Here's how the part is built. I have some questions about the finished solid (model axes, mm). Face numbers are marked on the shaded views. A direction names the side the tool comes from. Give positions to 0.01 mm unless a question says otherwise; leave off trailing zeros. Loops run counter-clockwise (first coordinate to the right, second up) from the corner with the lowest first, then second, coordinate; pieces in that order, holes last.
Q1. If we section it at D-D (z = 0): Give the number of separate pieces and of enclosed holes in the cut face, plus the area to 3 significant figures.
Q2. Will these pins go through, and if not, where does the flat tip stop? P1, Ø1.3, axis at x = 33, z = -56.5, coming from the +Y side; P2, Ø4, axis at x = -28, z = 35.5, coming from the +Y side; P3, Ø16.5, axis at x = 56.5, y = 13.5, coming from the -Z side.
Q3. If we section it at A-A (z = -35.5): Please give me the cut outline in (x, y).
Q4. We'd pull the mould along Y, two halves only. Please class the marked faces 1, 2 and 3: +Y half, -Y half, draft (parallel to the pull), parting line (faces both ways), or undercut.
Q5. For the marked faces 4, 5 and 6, which set-ups out of +Z, -Z, +X, -X, +Y, -Y let a thin tool reach every point of the face, with its end or its side?
Q6. I need wall thicknesses on line 1 (Z direction, x = 68, y = 27); line 2 (Z direction, x = -14, y = 16); line 3 (Y direction, x = 53, z = -8). Which ranges of each line are inside material? Lowest first, please.
Q7. If we section it at C-C (y = 11.5): Please give me the cut outline in (x, z), plus the area to 3 significant figures.
Q8. If we section it at B-B (x = 13): Please give me the cut outline in (y, z).
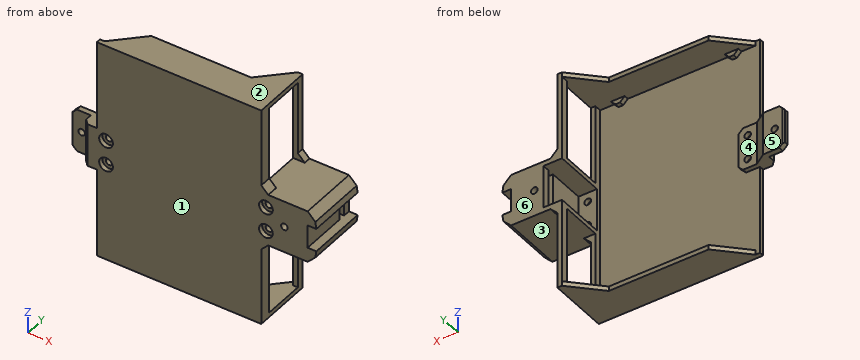
from build123d import *

# Parameters (mm, degrees)
SKETCH3_W                                       = 90.422573022
SKETCH3_H                                       = 121.412
BOSS_EXTRUDE4_DEPTH                             = 2.54
BOSS_EXTRUDE5_DEPTH                             = 30.48
CUT_EXTRUDE2_DEPTH                              = 122.412
BOSS_EXTRUDE6_DEPTH                             = 33.02
SKETCH9_W                                       = 10.16
SKETCH9_H                                       = 23.622
CUT_EXTRUDE3_DEPTH                              = 27.94
BOSS_EXTRUDE7_DEPTH                             = 2.54
SKETCH12_W                                      = 23.622
SKETCH12_H                                      = 3.81
CUT_EXTRUDE4_DEPTH                              = 10.16
SKETCH13_W                                      = 12.7
SKETCH13_H                                      = 3.81
CUT_EXTRUDE5_DEPTH                              = 13.461069207
BOSS_EXTRUDE9_REACH                             = 62.706
BOSS_EXTRUDE9_DIRECTION_2_REACH                 = 62.706
CBORE_FOR_6_PAN_HEAD_MACHINE_SCREW1_D           = 3.6576
CBORE_FOR_6_PAN_HEAD_MACHINE_SCREW1_CBORE_D     = 7.54126
CBORE_FOR_6_PAN_HEAD_MACHINE_SCREW1_CBORE_DEPTH = 2.4638
F_6_CLEARANCE_HOLE1_D                           = 3.6576
SKETCH21_W                                      = 43.815
SKETCH21_H                                      = 22.86
CUT_EXTRUDE6_DEPTH                              = 33.781069207
CHAMFER1_SIZE                                   = 2.54
CHAMFER2_SIZE                                   = 3.81
SKETCH22_W                                      = 17.78
SKETCH22_H                                      = 23.622
CUT_EXTRUDE7_DEPTH                              = 0.8
CHAMFER3_SIZE                                   = 0.8


with BuildPart() as part:
    # Sketch3 → Boss-Extrude4 (new body)
    with BuildSketch(Plane(origin=(0, 0, 0), x_dir=(1, 0, 0), z_dir=(0, 1, 0))):
        Rectangle(SKETCH3_W, SKETCH3_H)
    extrude(amount=BOSS_EXTRUDE4_DEPTH)

    # Sketch6 → Boss-Extrude5 (add)
    with BuildSketch(Plane(origin=(0, 2.54, 0), x_dir=(1, 0, 0), z_dir=(0, 1, 0))):
        Polygon((45.211286511, -60.706), (45.211286511, 60.706), (-45.211286511, 60.706), (-45.211286511, 58.166), (42.671286511, 58.166), (42.671286511, -58.166), (-45.211286511, -58.166), (-45.211286511, -60.706), align=None)
    extrude(amount=BOSS_EXTRUDE5_DEPTH)

    # Sketch7 → Cut-Extrude2 (cut, through all)
    with BuildSketch(Plane.XY.offset(60.706)):
        Polygon((-42.671286511, 2.54), (-27.431286511, 17.78), (27.431286511, 17.78), (42.671286511, 33.02), (-45.211286511, 33.02), (-45.211286511, 2.54), align=None)
    extrude(amount=-CUT_EXTRUDE2_DEPTH, mode=Mode.SUBTRACT)

    # Sketch8 → Boss-Extrude6 (add)
    with BuildSketch(Plane(origin=(0, 0, 0), x_dir=(1, 0, 0), z_dir=(0, 1, 0))):
        Polygon((45.211286511, 14.351), (70.694027546, 14.351), (74.922106204, 10.122921342), (75.452355719, 6.35), (70.677155719, 6.35), (70.677155719, -6.35), (75.452355719, -6.35), (74.922106204, -10.122921342), (70.694027546, -14.351), (45.211286511, -14.351), align=None)
    extrude(amount=BOSS_EXTRUDE6_DEPTH)

    # Sketch9 → Cut-Extrude3 (cut)
    with BuildSketch(Plane(origin=(0, 33.02, 0), x_dir=(1, 0, 0), z_dir=(0, 1, 0))):
        with Locations((47.751286511, 0)):
            Rectangle(SKETCH9_W, SKETCH9_H)
    extrude(amount=-CUT_EXTRUDE3_DEPTH, mode=Mode.SUBTRACT)

    # Sketch11 → Boss-Extrude7 (add)
    with BuildSketch(Plane(origin=(0, 2.54, 0), x_dir=(1, 0, 0), z_dir=(0, 1, 0))):
        Polygon((35.051286511, 58.166), (27.431286511, 58.166), (29.971286511, 55.626), (32.511286511, 55.626), align=None)
        Polygon((-29.971286511, 55.626), (-32.511286511, 55.626), (-35.051286511, 58.166), (-27.431286511, 58.166), align=None)
        Polygon((29.971286511, -55.626), (32.511286511, -55.626), (35.051286511, -58.166), (27.431286511, -58.166), align=None)
        Polygon((-27.431286511, -58.166), (-29.971286511, -55.626), (-32.511286511, -55.626), (-35.051286511, -58.166), align=None)
    extrude(amount=BOSS_EXTRUDE7_DEPTH)

    # Sketch12 → Cut-Extrude4 (cut)
    with BuildSketch(Plane.ZY.offset(-52.831286511)):
        with Locations((0, 27.305)):
            Rectangle(SKETCH12_W, SKETCH12_H)
    extrude(amount=-CUT_EXTRUDE4_DEPTH, mode=Mode.SUBTRACT)

    # Sketch13 → Cut-Extrude5 (cut, through all)
    with BuildSketch(Plane.ZY.offset(-62.991286511)):
        with Locations((0, 27.305)):
            Rectangle(SKETCH13_W, SKETCH13_H)
    extrude(amount=-CUT_EXTRUDE5_DEPTH, mode=Mode.SUBTRACT)

    # Boss-Extrude9: up to this face of the body (flat: up to its plane)
    boss_extrude9_end = Plane(part.part.faces().sort_by_distance((48.970486511, 20.0406, -11.811))[0])
    # Sketch15 → Boss-Extrude9 (add, up to the picked face)
    with BuildSketch(Plane.XY, mode=Mode.PRIVATE) as boss_extrude9_sk1:
        Polygon((-62.991286511, 10.16), (-52.831286511, 10.16), (-45.211286511, 5.08), (-35.051286511, 5.08), (-35.051286511, 2.54), (-45.211286511, 2.54), (-45.211286511, 0), (-52.831286511, 0), (-52.831286511, 6.35), (-62.991286511, 6.35), align=None)
    boss_extrude9_tool1 = split(extrude(boss_extrude9_sk1.sketch, amount=-BOSS_EXTRUDE9_REACH, mode=Mode.PRIVATE), bisect_by=boss_extrude9_end, keep=Keep.BOTH, mode=Mode.PRIVATE)
    add(boss_extrude9_tool1.solids().sort_by_distance((-50.157602, 5.280526, 0))[0])

    # Boss-Extrude9 direction 2: up to this face of the body (flat: up to its plane)
    boss_extrude9_direction_2_end = Plane(part.part.faces().sort_by_distance((48.970486511, 20.0406, 11.811))[0])
    # Sketch15 → Boss-Extrude9 direction 2 (add, up to the picked face)
    with BuildSketch(Plane.XY, mode=Mode.PRIVATE) as boss_extrude9_direction_2_sk1:
        Polygon((-62.991286511, 10.16), (-52.831286511, 10.16), (-45.211286511, 5.08), (-35.051286511, 5.08), (-35.051286511, 2.54), (-45.211286511, 2.54), (-45.211286511, 0), (-52.831286511, 0), (-52.831286511, 6.35), (-62.991286511, 6.35), align=None)
    boss_extrude9_direction_2_tool1 = split(extrude(boss_extrude9_direction_2_sk1.sketch, amount=BOSS_EXTRUDE9_DIRECTION_2_REACH, mode=Mode.PRIVATE), bisect_by=boss_extrude9_direction_2_end, keep=Keep.BOTH, mode=Mode.PRIVATE)
    add(boss_extrude9_direction_2_tool1.solids().sort_by_distance((-50.157602, 5.280526, 0))[0])

    # CBORE for #6 Pan Head Machine Screw1 (through all)
    with Locations(Plane(origin=(0, 0, 0), x_dir=(-1, 0, 0), z_dir=(0, -1, 0))):
        with Locations((-47.751286511, 6.731), (-47.751286511, -6.731), (40.131286511, 6.731), (40.131286511, -6.731)):
            CounterBoreHole(CBORE_FOR_6_PAN_HEAD_MACHINE_SCREW1_D / 2, CBORE_FOR_6_PAN_HEAD_MACHINE_SCREW1_CBORE_D / 2, CBORE_FOR_6_PAN_HEAD_MACHINE_SCREW1_CBORE_DEPTH)

    # #6 Clearance Hole1 (through all)
    with Locations(Plane(origin=(0, 33.02, 0), x_dir=(1, 0, 0), z_dir=(0, 1, 0))):
        with Locations((-57.911286511, 0), (57.911286511, 0)):
            Hole(F_6_CLEARANCE_HOLE1_D / 2)

    # Sketch21 → Cut-Extrude6 (cut, through all)
    with BuildSketch(Plane.ZY.offset(-42.671286511)):
        with Locations((-36.2585, 17.78)):
            Rectangle(SKETCH21_W, SKETCH21_H)
        with Locations((36.2585, 17.78)):
            Rectangle(SKETCH21_W, SKETCH21_H)
    extrude(amount=-CUT_EXTRUDE6_DEPTH, mode=Mode.SUBTRACT)

    # Chamfer1
    chamfer1_edges = [part.edges().sort_by_distance(p)[0] for p in [
        (-52.831286511, 0, 0),
        (-35.051286511, 3.81, -11.811),
        (-62.991286511, 8.255, -11.811),
        (-62.991286511, 8.255, 11.811),
        (-35.051286511, 3.81, 11.811),
    ]]
    chamfer(chamfer1_edges, length=CHAMFER1_SIZE)

    # Chamfer2
    chamfer2_edges = [part.edges().sort_by_distance(p)[0] for p in [
        (45.211286511, 3.175, -14.351),
        (45.211286511, 3.175, 14.351),
        (45.211286511, 31.115, -14.351),
        (45.211286511, 31.115, 14.351),
    ]]
    chamfer(chamfer2_edges, length=CHAMFER2_SIZE)

    # Sketch22 → Cut-Extrude7 (cut)
    with BuildSketch(Plane(origin=(0, 10.16, 0), x_dir=(1, 0, 0), z_dir=(0, 1, 0))):
        with Locations((-54.101286511, 0)):
            Rectangle(SKETCH22_W, SKETCH22_H)
    extrude(amount=-CUT_EXTRUDE7_DEPTH, mode=Mode.SUBTRACT)

    # Chamfer3
    chamfer3_edges = [part.edges().sort_by_distance(p)[0] for p in [
        (-62.991286511, 9.36, 0),
    ]]
    chamfer(chamfer3_edges, length=CHAMFER3_SIZE)


solid = part.part
Check sheet entries:
1. separate pieces: 5
1. enclosed holes: 0
1. area: 789 mm2
2. P1: stops at y = 5.08
2. P2: stops at y = 2.54
2. P3: stops at z = -14.35
3. outline: (-45.21, 0) - (45.21, 0) - (45.21, 6.35) - (42.67, 6.35) - (42.67, 2.54) - (-45.21, 2.54) - close; (42.67, 29.21) - (45.21, 29.21) - (45.21, 33.02) - (42.67, 33.02) - close
4. face 1: -Y half
4. face 2: draft
4. face 3: undercut
5. face 4: +Y
5. face 5: +Z, -Z, -X, +Y
5. face 6: +Z, -Z, +X, -X, +Y
6. line 1: z = -14.35 to -6.35, 6.35 to 14.35
6. line 2: z = -60.71 to -58.17, 58.17 to 60.71
6. line 3: y = 0 to 25.4, 29.21 to 33.02
7. outline: (-33.71, -60.71) - (45.21, -60.71) - (45.21, -58.17) - (-33.71, -58.17) - close; (-33.71, 58.17) - (45.21, 58.17) - (45.21, 60.71) - (-33.71, 60.71) - close; (42.67, -14.35) - (70.69, -14.35) - (74.92, -10.12) - (75.45, -6.35) - (70.68, -6.35) - (70.68, 6.35) - (75.45, 6.35) - (74.92, 10.12) - (70.69, 14.35) - (42.67, 14.35) - (42.67, 11.81) - (52.83, 11.81) - (52.83, -11.81) - (42.67, -11.81) - close; hole circle Ø3.66 at (57.91, 0)
7. area: 1,010 mm2
8. outline: (0, -60.71) - (17.78, -60.71) - (17.78, -58.17) - (2.54, -58.17) - (2.54, 58.17) - (17.78, 58.17) - (17.78, 60.71) - (0, 60.71) - close
